```python
from build123d import *

# Parameters (mm, degrees)
F1_DEPTH      = 20
F2_W          = 7
F2_H          = 20
F3_DEPTH      = 2
F5_DEPTH      = 6
F6_W          = 3
F6_H          = 6
F7_DEPTH      = 25
F8_DEPTH      = 3
F12_DEPTH     = 2
F13_DEPTH     = 11
F14_T4_DEPTH  = 29
F14_T10_DEPTH = 28
F14_T17_DEPTH = 38.2867319519
F14_T24_DEPTH = 39.2867319519
F15_T1_DEPTH  = 61.1449358039
F15_T3_DEPTH  = 60.1449358039
F16_DEPTH     = 1
F17_SIZE      = 6
F20_D         = 2.85
F20_ON_F18_D  = 2.85


# Not quite as in the source:
# - a fillet or chamfer that OpenCascade refuses, or shapes differently, is made with other operations: its cross-section is extruded or revolved along the edge and cut away or added


with BuildPart() as f1:
    # F0 (on Top) → F1 (new body)
    with BuildSketch(Plane.XY):
        Polygon((-3.1551690071, 9.1141472052), (-12.1551690071, 9.1141472052), (-12.1551690071, -0.8858527948), (-3.1551690071, -0.8858527948), (-3.1551690071, 2.1141472052), (-9.1551690071, 2.1141472052), (-9.1551690071, 6.1141472052), (-3.1551690071, 6.1141472052), align=None)
    extrude(amount=F1_DEPTH)

    # F2 (on face) → F3 (join)
    with BuildSketch(Plane(origin=(-12.1551690071, 0, 0), x_dir=(0, -1, 0), z_dir=(-1, 0, 0))):
        with Locations((-5.6141472052, 10)):
            Rectangle(F2_W, F2_H)
    extrude(amount=F3_DEPTH)

    # F4 (on face) → F5 (join)
    with BuildSketch(Plane.XY.offset(20)):
        Polygon((-12.1345976368, 9.1141472052), (-12.1551690071, 2.1141472052), (-12.1551690071, -0.8858527948), (-9.1551690071, -0.8858527948), (-9.1551690071, 2.1141472052), (-9.1551690071, 6.1141472052), (-9.1551690071, 9.1141472052), align=None)
    extrude(amount=F5_DEPTH)

    # F6 (on face) → F7 (join)
    with BuildSketch(Plane.YZ.offset(-9.1551690071)):
        with Locations((7.6141472052, 23)):
            Rectangle(F6_W, F6_H)
        with Locations((0.6141472052, 23)):
            Rectangle(F6_W, F6_H)
        Polygon((-0.8858527948, 26), (2.1141472052, 26), (6.1141472052, 26), (9.1141472052, 26), (9.1141472052, 29), (-0.8858527948, 29), align=None)
    extrude(amount=F7_DEPTH)

    # F8 (add): a face of the model
    f8_faces = [f1.faces().sort_by_distance(p)[0] for p in [
        (-10.6515768532, 4.1077318265, 26),
    ]]
    extrude(f8_faces, amount=F8_DEPTH)

    # F9: union 

    # F10: union 

    # F11 (on face) → F12 (join)
    with BuildSketch(Plane.XY.offset(29)):
        Polygon((-12.1345976368, 9.1141472052), (-12.1551690071, 2.1141472052), (15.8448309929, 2.1141472052), (15.8448309929, 9.1141472052), align=None)
    extrude(amount=F12_DEPTH)

    # F4 (on face) → F13 (join)
    with BuildSketch(Plane.XY.offset(20)):
        Polygon((-14.1551690071, 2.1141472052), (-12.1551690071, 2.1141472052), (-12.1345976368, 9.1141472052), (-14.1551690071, 9.1141472052), align=None)
    extrude(amount=F13_DEPTH)

    # F14: chamfer of 4 on 2 edges, made by hand


with BuildPart() as f14_tool2:
    # F14_s3 → F14_t4 (new body)
    with BuildSketch(Plane.XY):
        Polygon((-12.1551690071, -1.8858527948), (-16.1551690071, 2.1141472052), (-12.1551690071, 2.1141472052), align=None)
    extrude(amount=F14_T4_DEPTH)

    split(bisect_by=Plane.XZ.offset(0.8858527948), keep=Keep.BOTTOM)

    split(bisect_by=Plane.YZ.offset(-14.1551690071), keep=Keep.TOP)


with BuildPart() as f1_1:
    add(f1.part)

    # F14_t1: union F14_tool2
    add(f14_tool2.part)


with BuildPart() as f14_tool8:
    # F14_s9 → F14_t10 (new body)
    with BuildSketch(Plane.YZ.offset(-12.1551690071)):
        Polygon((-1.8858527948, 29), (2.1141472052, 33), (2.1141472052, 29), align=None)
    extrude(amount=F14_T10_DEPTH)

    split(bisect_by=Plane.XZ.offset(0.8858527948), keep=Keep.BOTTOM)

    split(bisect_by=Plane.XY.offset(31), keep=Keep.BOTTOM)


with BuildPart() as f1_2:
    add(f1_1.part)

    # F14_t7: union F14_tool8
    add(f14_tool8.part)


with BuildPart() as f14_tool15:
    # F14_s16 → F14_t17 (new body)
    with BuildSketch(Plane.YZ.offset(-22.4419009589)):
        Polygon((-1.8858527948, 29), (2.1141472052, 33), (2.1141472052, 29), align=None)
    extrude(amount=F14_T17_DEPTH)

    split(bisect_by=Plane.XZ.offset(0.8858527948), keep=Keep.BOTTOM)

    split(bisect_by=Plane.YZ.offset(-12.1551690071), keep=Keep.BOTTOM)

    split(bisect_by=Plane.YZ.offset(-14.1551690071), keep=Keep.TOP)

    split(bisect_by=Plane.XY.offset(31), keep=Keep.BOTTOM)


with BuildPart() as f14_tool22:
    # F14_s23 → F14_t24 (new body)
    with BuildSketch(Plane.XY):
        Polygon((-12.1551690071, -1.8858527948), (-16.1551690071, 2.1141472052), (-12.1551690071, 2.1141472052), align=None)
    extrude(amount=F14_T24_DEPTH)

    split(bisect_by=Plane.XZ.offset(0.8858527948), keep=Keep.BOTTOM)

    split(bisect_by=Plane.XY.offset(29), keep=Keep.TOP)

    split(bisect_by=Plane.YZ.offset(-14.1551690071), keep=Keep.TOP)

    split(bisect_by=Plane.XY.offset(31), keep=Keep.BOTTOM)


with BuildPart() as f14_tool15_1:
    add(f14_tool15.part)

    # F14_t29: intersect F14_tool22
    add(f14_tool22.part, mode=Mode.INTERSECT)


with BuildPart() as f1_3:
    add(f1_2.part)

    # F14_t13: union F14_tool15
    add(f14_tool15_1.part)

    # F15: chamfer of 4 x 6 on 2 edges, made by hand

    # F15_s2 → F15_t1 (cut)
    with BuildSketch(Plane.XY.offset(-15.5724679019)):
        Polygon((-9.1551690071, -0.8858527948), (-17.3978096942, 3.3567878923), (-13.1551690071, -0.8858527948), align=None)
    extrude(amount=F15_T1_DEPTH, mode=Mode.SUBTRACT)

    # F15_s4 → F15_t3 (cut)
    with BuildSketch(Plane.YZ.offset(-28.7276369091)):
        Polygon((-0.8858527948, 26), (3.3567878923, 34.2426406871), (-0.8858527948, 30), align=None)
    extrude(amount=F15_T3_DEPTH, mode=Mode.SUBTRACT)

    # F16 (add): a face of the model
    f16_faces = [f1_3.faces().sort_by_distance(p)[0] for p in [
        (15.8448309929, 6.2628078927, 23),
    ]]
    extrude(f16_faces, amount=F16_DEPTH)

    # F17
    f17_edges = [f1_3.edges().sort_by_distance(p)[0] for p in [
        (-3.155169, 0.614147, 0),
        (-3.155169, 7.614147, 0),
        (16.844831, 0.614147, 20),
        (16.844831, 7.614147, 20),
    ]]
    chamfer(f17_edges, length=F17_SIZE)

    # F20 (through all)
    with Locations(Plane(origin=(0, 0, 0), x_dir=(1, 0, 0), z_dir=(0, 0, -1))):
        with Locations((-13.6551690071, -4.6141472052)):
            Hole(F20_D / 2)

    # F20 on F18 (through all)
    with Locations(Plane.YZ.offset(16.8448309929)):
        with Locations((4.6141472052, 28.7)):
            Hole(F20_ON_F18_D / 2)


solid = f1_3.part
```
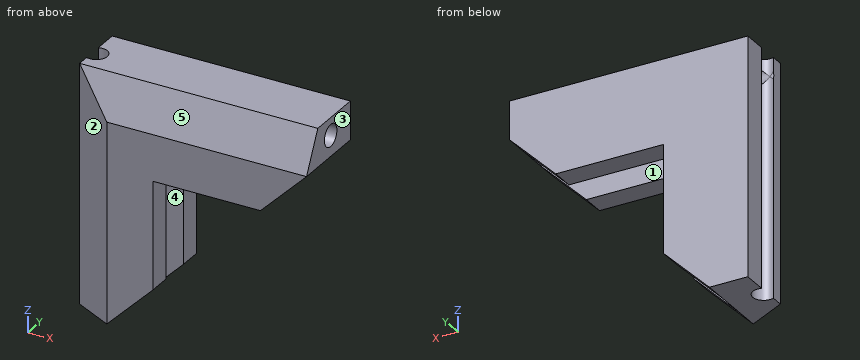
Read the model definition and answer for the solid it produces. Units are mm, in the model's axes. Face numbers are marked on the shaded views. A direction names the side the tool comes from. Coordinates: 2 decimals unless noted, no trailing zeros. Loops run counter-clockwise (first coordinate to the right, second up) from the corner with the lowest first, then second, coordinate; pieces in that order, holes last. Notation, with made-up numbers: (42.5, 48) -> (74.5, 48) arc R32 ccw to (74.5, 75) -> close; hole circle Ø2 at (-34, 3.25). An arc over 180 degrees is marked (long way). Return JSON: item names as keys, results as strings.
Item 1: Find section A-A (x = 4.5). Determine the outline of the cut face in (y, z) (3 decimals).
Answers:
{"outline": "(-0.886, 20) -> (2.114, 20) -> (2.114, 26) -> (6.114, 26) -> (6.114, 20) -> (9.114, 20) -> (9.114, 31) -> (1.688, 31) -> (-0.886, 26) -> close; hole circle Ø2.85 at (4.614, 28.7)"}
Item 2: For the marked faces 1 and 2, determine the directions among +Z, -Z, +X, -X, +Y, -Y from which every point of the face is accessible in a straight line to the end or side of a thin tool.
Answers:
{"face 1": "-Z, +X", "face 2": "+Z, -Z, -X, -Y"}
Item 3: For a pull along Y with two mould halves and no side action, classify the marked faces 3, 4 and 5 as +Y half, -Y half, draft (parallel to the pull), parting line (faces both ways), or undercut.
Answers:
{"face 3": "draft", "face 4": "undercut", "face 5": "-Y half"}
Item 4: Flat-ended cylindrical pins translate along their axes: P1, Ø2.5, axis at y = 8, z = 11.5, coming from the +X side; P2, Ø3, axis at x = -0.5, y = 5, coming from the -Z side; P3, Ø3.5, axis at x = -13.66, y = 4.61, coming from the +Z side; P4, Ø1, axis at y = 0.5, z = 25, coming from the -X side. Find the tip coordinate at first contact, or state that the pin passes through.
Answers:
{"P1": "stops at x = -3.16", "P2": "stops at z = 20", "P3": "stops at z = 31", "P4": "stops at x = -12.82"}
Item 5: Find section D-D (z = 18.5). Determine the outline of the cut face in (x, y) (3 decimals).
Answers:
{"outline": "(-14.155, 1.688) -> (-9.155, -0.886) -> (-3.155, -0.886) -> (-3.155, 2.114) -> (-9.155, 2.114) -> (-9.155, 6.114) -> (-3.155, 6.114) -> (-3.155, 9.114) -> (-14.155, 9.114) -> (-14.155, 5.949) arc R1.425 cw (long way) to (-14.155, 3.28) -> close"}
Item 6: Find section C-C (z = 25). Determine the outline of the cut face in (x, y) (3 decimals).
Answers:
{"outline": "(-14.155, 1.688) -> (-9.155, -0.886) -> (15.845, -0.886) -> (15.845, 2.114) -> (-9.155, 2.114) -> (-9.155, 6.114) -> (15.845, 6.114) -> (15.845, 9.114) -> (-14.155, 9.114) -> (-14.155, 5.949) arc R1.425 cw (long way) to (-14.155, 3.28) -> close"}
Item 7: Find section B-B (y = 3.75). Determine the outline of the cut face in (x, z).
Answers:
{"outline": "(-12.52, 0) -> (-9.16, 0) -> (-9.16, 26) -> (16.84, 26) -> (16.84, 27.57) -> (-12.52, 27.57) -> close; (-12.52, 29.83) -> (16.84, 29.83) -> (16.84, 31) -> (-12.52, 31) -> close"}
Item 8: Find the intervals of material crossed by probe 1 along Y at (x, z) = (-3.5, 16); probe 2 along X at (y, z) = (7.25, 18.5); probe 3 along Z at (x, y) = (-3.5, 3), in increasing order.
Answers:
{"probe 1": "y = -0.89 to 2.11, 6.11 to 9.11", "probe 2": "x = -14.16 to -3.16", "probe 3": "z = 26 to 31"}
